For this review, take the finished solid that the model builds, in its own axes (mm). A direction names the side the tool comes from. Coordinates: 2 decimals unless noted, no trailing zeros. Order: outer loops, then holes, each group sorted by start corner. A loop starts at its lowest first (then second) coordinate and runs counter-clockwise, first axis right, second up. Notation, with made-up numbers: (-22.5, 43.5) - (17.5, 43.5) arc R5 cw to (17.5, 51.5) - close; hole circle Ø9 at (63, -35). An arc over 180 degrees is marked (long way). One line per item, written item: value. Start each with the question number.
(1) Mouldability with a two-part tool opening along Y and no side actions: class faces 6 (the cylindrical face through (-270.31, -343.54, 4.52)), 7 (the flat face through (-267, -338, 21)), 8 (the cylindrical face through (-273.574, -348.589, 5.535)) as released by +Y, released by -Y, zero draft, split by the parting line, or undercut.
(2) Clearance check with flat-ended pins moving along their axes: pin 1 (2.5 mm diameter, centred on x = -271.5, y = -338, fed in from +Z); pin 2 (1 mm diameter, centred on y = -334, z = 26, fed in from +X); pin 3 (2.5 mm diameter, centred on x = -271, y = -334.32, fed in from +Z); pin 4 (1.5 mm diameter, centred on y = -345, z = 24.5, fed in from -X). State where each tip first meets the part, or that it passes through.
(3) Consider section D-D on y = -343. Write out the cut boundary in (x, z).
(4) To check wall thickness, follow line 1 along Z through (x, y) = (-252.5, -346); line 2 along X through (y, z) = (-334.25, 6.5); line 3 along Y through (x, z) = (-271, 4). State the ranges of each line that lie inside material, in increasing order.
(5) Consider section C-C on x = -271. Write out the cut boundary in (y, z).
(6) Consider section A-A on x = -259.25. Write out the cut boundary in (y, z), then the cut area to 3 significant figures.
(7) Consider section B-B on y = -337.25. Write out the cut boundary in (x, z), then the cut area to 3 significant figures.
(8) For faces 1 (the flat face through (-255, -338, 28)), 2 (the flat face through (-259, -338, 33)), 3 (the flat face through (-263, -338, 3)), 4 (the flat face through (-271, -338, 6)), 5 (the flat face through (-267.5, -338.1, 8)), list the 3-axis set-ups (+Z, -Z, +X, -X, +Y, -Y) from which the entire face can be reached by the end or side of a thin tool; tool diameter is ignored.
```python
from build123d import *

# Parameters (mm, degrees)
SKETCH010_W     = 25
SKETCH010_H     = 23.658539
PAD002_DEPTH    = 30
SKETCH011_W     = 17.384644
SKETCH011_H     = 39.730011
POCKET008_DEPTH = 25
SKETCH012_R     = 1.5
POCKET009_DEPTH = 5.001
POCKET010_DEPTH = 2
SKETCH014_W     = 12.358228
SKETCH014_H     = 3.3
POCKET011_DEPTH = 23.659539
FILLET004_R     = 5


with BuildPart() as part:
    # Sketch010 → Pad002 (new body)
    with BuildSketch(Plane.XY):
        with Locations((-262.5, -338.263442)):
            Rectangle(SKETCH010_W, SKETCH010_H)
    extrude(amount=PAD002_DEPTH)

    # Sketch011 (on Face6 of Pad002) → Pocket008 (cut)
    with BuildSketch(Plane.XY.offset(30)):
        with Locations((-275.692322, -336.624282)):
            Rectangle(SKETCH011_W, SKETCH011_H)
    extrude(amount=-POCKET008_DEPTH, mode=Mode.SUBTRACT)

    # Sketch012 (on Face6 of Pocket008) → Pocket009 (cut, through all)
    with BuildSketch(Plane.XY.offset(5)):
        with Locations((-271, -334.320353)):
            Circle(SKETCH012_R)
        with Locations((-271, -342.206532)):
            Circle(SKETCH012_R)
    extrude(amount=-POCKET009_DEPTH, mode=Mode.SUBTRACT)

    # Sketch013 (on Face6 of Pocket009) → Pocket010 (cut)
    with BuildSketch(Plane.XY.offset(5)):
        with BuildLine():
            ThreePointArc((-268, -334.320353), (-271, -331.320353), (-274, -334.320353))
            Line((-274, -334.320353), (-274, -342.206532))
            ThreePointArc((-274, -342.206532), (-271, -345.206532), (-268, -342.206532))
            Line((-268, -334.320353), (-268, -342.206532))
        make_face()
    extrude(amount=-POCKET010_DEPTH, mode=Mode.SUBTRACT)

    # Sketch014 (on Face1 of Pocket010) → Pocket011 (cut, through all)
    with BuildSketch(Plane.XZ.offset(350.092712)):
        with Locations((-254.010886, 23.35)):
            Rectangle(SKETCH014_W, SKETCH014_H)
    extrude(amount=-POCKET011_DEPTH, mode=Mode.SUBTRACT)

    # Fillet004
    fillet004_edges = [part.edges().sort_by_distance(p)[0] for p in [
        (-275, -326.434173, 2.5),
        (-275, -350.092712, 2.5),
    ]]
    fillet(fillet004_edges, radius=FILLET004_R)


with BuildPart() as part_1:
    # Body002 placement: moved
    add(part.part.moved(Location((0, 0, 3))))


solid = part_1.part
```
Geometry check:
1. face 6: undercut
1. face 7: zero draft
1. face 8: released by -Y
2. pin 1: stops at z = 6
2. pin 2: stops at x = -260.19
2. pin 3: passes through
2. pin 4: stops at x = -267
3. outline: (-275, 3) - (-272.27, 3) - (-272.27, 6) - (-273.89, 6) - (-273.89, 8) - (-275, 8) - close; (-269.73, 3) - (-250, 3) - (-250, 24.7) - (-260.19, 24.7) - (-260.19, 28) - (-250, 28) - (-250, 33) - (-267, 33) - (-267, 8) - (-268.11, 8) - (-268.11, 6) - (-269.73, 6) - close
4. line 1: z = 3 to 24.7, 28 to 33
4. line 2: x = -275 to -274, -268 to -250
4. line 3: y = -349.99 to -343.71, -340.71 to -335.82, -332.82 to -326.54
5. outline: (-349.99, 3) - (-343.71, 3) - (-343.71, 6) - (-345.21, 6) - (-345.21, 8) - (-349.99, 8) - close; (-340.71, 3) - (-335.82, 3) - (-335.82, 6) - (-340.71, 6) - close; (-332.82, 3) - (-326.54, 3) - (-326.54, 8) - (-331.32, 8) - (-331.32, 6) - (-332.82, 6) - close
6. outline: (-350.09, 3) - (-326.43, 3) - (-326.43, 24.7) - (-350.09, 24.7) - close; (-350.09, 28) - (-326.43, 28) - (-326.43, 33) - (-350.09, 33) - close
6. area: 632 mm^2
7. outline: (-275, 3) - (-250, 3) - (-250, 24.7) - (-260.19, 24.7) - (-260.19, 28) - (-250, 28) - (-250, 33) - (-267, 33) - (-267, 8) - (-268, 8) - (-268, 6) - (-274, 6) - (-274, 8) - (-275, 8) - close
7. area: 504 mm^2
8. face 1: +X, +Y, -Y
8. face 2: +Z, +X, -X, +Y, -Y
8. face 3: -Z, +X, -X, +Y, -Y
8. face 4: +Z
8. face 5: +Z, -X, +Y, -Y
